Autodesk Inventor part; units mm, degrees
ref_plane "YZ Plane" through (0, 0, 0) normal (1, 0, 0) x (0, 1, 0)
ref_plane "XZ Plane" through (0, 0, 0) normal (0, 1, 0) x (-1, 0, 0)
ref_plane "XY Plane" through (0, 0, 0) normal (0, 0, 1) x (1, 0, 0)
sketch "Sketch1" plane through (0, 0, 0) normal (0, 0, 1) x (1, 0, 0)
  line L0 (-25.4, -304.8) -> (25.4, -304.8)
  line L1 (25.4, -304.8) -> (25.4, 304.8)
  line L2 (25.4, 304.8) -> (-25.4, 304.8)
  line L3 (-25.4, 304.8) -> (-25.4, -304.8)
  line L4 (-25.4, -304.8) -> (25.4, 304.8) construction
  line L5 (25.4, -304.8) -> (-25.4, 304.8) construction
  point P0 (0, 0)
  dimension "d0" = 50.8
  dimension "d1" = 609.6
extrude "Extrusion1" add sketch "Sketch1" along normal mid plane 25.4
sketch "Sketch2" plane through (0, 0, 0) normal (0, 1, 0) x (-1, 0, 0)
  line L0 (-22.225, 9.525) -> (-22.225, -9.525)
  line L1 (-22.225, -9.525) -> (22.225, -9.525)
  line L2 (22.225, -9.525) -> (22.225, 9.525)
  line L3 (22.225, 9.525) -> (-22.225, 9.525)
  line L4 (-22.225, 9.525) -> (22.225, -9.525) construction
  line L5 (-22.225, -9.525) -> (22.225, 9.525) construction
  line L6 (25.4, -12.7) -> (25.4, 12.7)
  line L7 (25.4, 12.7) -> (-25.4, 12.7)
  point P0 (0, 0)
  dimension "d4" = 3.175
  dimension "d5" = 3.175
extrude "Extrusion2" cut sketch "Sketch2" along normal through all both and the other way through all
equation "\"d0\" = width"
equation "\"d1\" = height"
equation "\"d2\" = depth"
equation "\"d4\" = wallThickness"
equation "\"d5\" = wallThickness"
equation "\"depth\" = 25.4"
equation "\"width\" = 50.8"
equation "\"height\" = 609.6"
equation "\"wallThickness\" = 3.175"
properties part number "1x2x24inAluminumExtrusion"
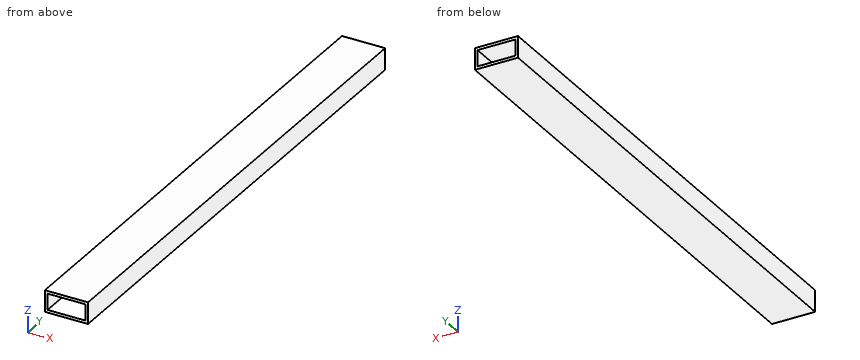
Read the model definition and answer for the solid it produces. Units are mm, in the model's axes. Give positions to 0.01 mm unless a question says otherwise; leave off trailing zeros. Order: outer loops, then holes, each group sorted by start corner. A loop starts at its lowest first (then second) coordinate and runs counter-clockwise, first axis right, second up.
(1) Find section A-A (z = 1.5). Give the vertices of the cut face in (x, y) (3 decimals), plus the area to 3 significant figures.
(2) Find section B-B (x = -10). Give the vertices of the cut face in (y, z) (3 decimals), plus the area to 3 significant figures.
(3) Straight lines are drawn through the part: L1, parallel to Z at x = 22, y = 58 (3 decimals); L2, parallel to X at y = -10, z = 6.5 (3 decimals). For each, find the intervals that lie inside material, in ascending order.
(4) Find section C-C (y = 167). Give the vertices of the cut face in (x, z) (3 decimals).
Result sheet:
1. outline: (-25.4, -304.8) - (-22.225, -304.8) - (-22.225, 304.8) - (-25.4, 304.8) - close; (22.225, -304.8) - (25.4, -304.8) - (25.4, 304.8) - (22.225, 304.8) - close
1. area: 3,870 mm2
2. outline: (-304.8, -12.7) - (304.8, -12.7) - (304.8, -9.525) - (-304.8, -9.525) - close; (-304.8, 9.525) - (304.8, 9.525) - (304.8, 12.7) - (-304.8, 12.7) - close
2. area: 3,870 mm2
3. L1: z = -12.7 to -9.525, 9.525 to 12.7
3. L2: x = -25.4 to -22.225, 22.225 to 25.4
4. outline: (-25.4, -12.7) - (25.4, -12.7) - (25.4, 12.7) - (-25.4, 12.7) - close; hole (-22.225, -9.525) - (22.225, -9.525) - (22.225, 9.525) - (-22.225, 9.525) - close
